Input: dimensioned drawing with shaded views. Units: mm. Origin: part minimum x, y, z. A direction names the side the tool comes from. Give positions to 0.01 mm unless a question says otherwise; leave off trailing zeros. Write each loop counter-clockwise with the first axis right and the second up, starting at its lowest first coordinate (ties: lowest second). Pieces come first, ordered by that corner, then holes.
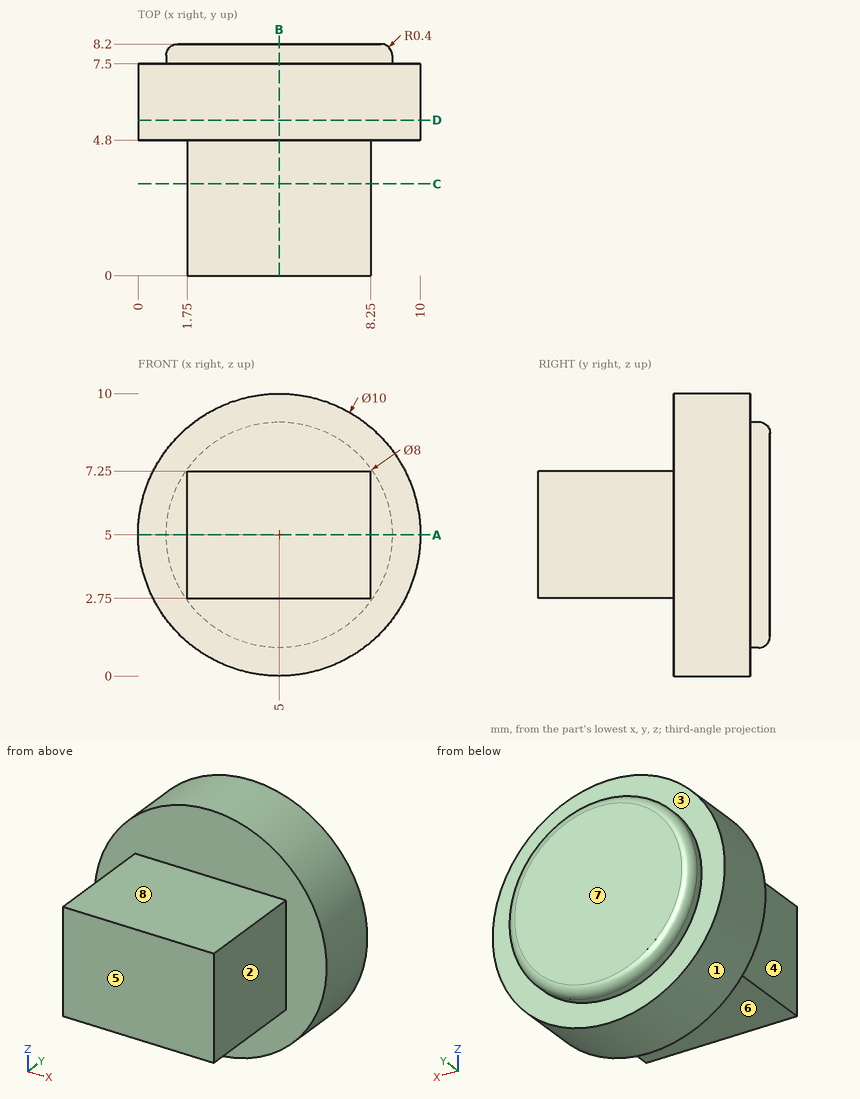
1. Cut plane C-C, the plane y = 3.25. Return the cut outline in (x, z).
2. Access query for the marked faces 1, 2, 3, 4 and 5. Directions: +Z, -Z, +X, -X, +Y, -Y. A direction counts if a zero-diameter tool reaches every point of the face in a straight line with its end or side. Return the directions, or none.
3. Mould query, pull axis Z, two halves, no side actions, for the marked faces 6, 7 and 8. Classes: +Z half, -Z half, draft (parallel to the pull), parting line (faces both ways), or undercut.
4. Line query: L1, parallel to Z at x = 6.5, y = 4; L2, parallel to Y at x = 4.5, z = 1.75; L3, parallel to Y at x = 7, z = 9.5. Output: solid intervals per line, ascending.
5. Cut plane B-B, the plane x = 5. Return the cut outline in (y, z), then the cut area to 3 significant figures.
6. Contact query for flat-ended pins moving along their axis: P1, Ø3.5, axis at y = 3, z = 5, coming from the +X side; P2, Ø1.5, axis at y = 7, z = 2.5, coming from the +X side; P3, Ø1.3, axis at y = 2, z = 6, coming from the -X side. Output: stop coordinate, or through.
7. Cut plane A-A, the plane z = 5. Return the cut outline in (x, y).
8. Cut plane D-D, the plane y = 5.5. Return the cut outline in (x, z).
Response values:
1. outline: (1.75, 2.75) - (8.25, 2.75) - (8.25, 7.25) - (1.75, 7.25) - close
2. face 1: +Y, -Y
2. face 2: +Z, -Z, +X, -Y
2. face 3: +Y
2. face 4: +Z, -Z, -X, -Y
2. face 5: +Z, -Z, +X, -X, -Y
3. face 6: -Z half
3. face 7: draft
3. face 8: +Z half
4. L1: z = 2.75 to 7.25
4. L2: y = 4.8 to 8.2
4. L3: y = 4.8 to 7.5
5. outline: (0, 2.75) - (4.8, 2.75) - (4.8, 0) - (7.5, 0) - (7.5, 1) - (7.8, 1) arc R0.4 ccw to (8.2, 1.4) - (8.2, 8.6) arc R0.4 ccw to (7.8, 9) - (7.5, 9) - (7.5, 10) - (4.8, 10) - (4.8, 7.25) - (0, 7.25) - close
5. area: 54.1 mm2
6. P1: stops at x = 8.25
6. P2: stops at x = 9.68
6. P3: stops at x = 1.75
7. outline: (0, 4.8) - (1.75, 4.8) - (1.75, 0) - (8.25, 0) - (8.25, 4.8) - (10, 4.8) - (10, 7.5) - (9, 7.5) - (9, 7.8) arc R0.4 ccw to (8.6, 8.2) - (1.4, 8.2) arc R0.4 ccw to (1, 7.8) - (1, 7.5) - (0, 7.5) - close
8. outline: circle Ø10 at (5, 5)
